Design review of the part built by this model. Coordinates are the model's own, in mm. Coordinates: 2 decimals unless noted, no trailing zeros. Loops run counter-clockwise (first coordinate to the right, second up) from the corner with the lowest first, then second, coordinate; pieces in that order, holes last. Notation, with made-up numbers: (68, -12.75) -> (110, -12.75) arc R22 cw to (110, 7.25) -> close; hole circle Ø6 at (-6, -17). An arc over 180 degrees is marked (long way). Use a Markdown table: item, result. Add a question column.
Q1. Take a section at D-D on z = 3. Write out the cut boundary in (x, y).
Q2. Take a section at B-B on x = -52.5. Write out the cut boundary in (y, z), plus the area to 3 significant figures.
Q3. Clearance check with a flat-ended pin moving along its axis: pin 1 Ø11.5 at (x, y) = (-50.8, 50.8) entering from -Z. State where the tip first meets the part, or that it passes through.
Q4. For probe 1 along Y at (x, z) = (-50.8, -3.5); probe 2 along X at (y, z) = (50.8, -20); probe 3 along Z at (x, y) = (6, 12), list the stretches that pass through material, from the lowest coordinate up.
Q5. Take a section at A-A on x = 0. Write out the cut boundary in (y, z).
Q6. Draft analysis for pull direction X (two halves, no side actions). For faces 1 (the face through (-1, 63.5, -13)), 2 (the face through (1, -1, -1.524)), 3 (the face through (63.5, -1, -14)), state which applies: pulls with the +X half, pulls with the -X half, needs draft (parallel to the pull), parting line crosses it, or undercut.
from build123d import *

# Parameters (mm, degrees)
F2_DEPTH = 63.5
F5_DEPTH = 50.8


with BuildPart() as f2:
    # F1 (on Front) → F2 (new body, symmetric)
    with BuildSketch(Plane.XZ):
        Polygon((-63.5, -32.291652), (63.5, -32.291652), (63.5, 5.808348), (0, 5.808348), (-63.5, 5.808348), align=None)
    extrude(amount=F2_DEPTH, both=True)

    # F0 (on Front) → F3 (revolve, cut)
    with BuildSketch(Plane.XZ):
        Polygon((38.1, -1.524), (50.8, 5.808348), (0, 5.808348), (0, -1.524), align=None)
    revolve(axis=Axis((0, 0, 2.142174), (0, 0, -1)), mode=Mode.SUBTRACT)

    # F4 (on Top) → F5 (cut, symmetric)
    with BuildSketch(Plane.XY):
        with BuildLine():
            ThreePointArc((-44.45, 50.8), (-55.290128, 55.290128), (-50.8, 44.45))
            Line((-50.8, 44.45), (-50.8, 50.8))
            Line((-50.8, 50.8), (-44.45, 50.8))
        make_face()
        with BuildLine():
            Line((-50.8, 50.8), (-50.8, 44.45))
            ThreePointArc((-50.8, 44.45), (-46.309872, 46.309872), (-44.45, 50.8))
            Line((-44.45, 50.8), (-50.8, 50.8))
        make_face()
    extrude(amount=F5_DEPTH, both=True, mode=Mode.SUBTRACT)


solid = f2.part
Answer list:
| question | item | result |
|---|---|---|
| 1 | outline | (-63.5, -63.5) -> (63.5, -63.5) -> (63.5, 63.5) -> (-63.5, 63.5) -> close; hole circle Ø12.7 at (-50.8, 50.8); hole circle Ø91.87 at (0, 0) |
| 2 | outline | (-63.5, -32.29) -> (44.68, -32.29) -> (44.68, 5.81) -> (-63.5, 5.81) -> close; (56.92, -32.29) -> (63.5, -32.29) -> (63.5, 5.81) -> (56.92, 5.81) -> close |
| 2 | area | 4,370 mm² |
| 3 | pin 1 | through |
| 4 | probe 1 | -63.5 to 44.45, 57.15 to 63.5 |
| 4 | probe 2 | -63.5 to -57.15, -44.45 to 63.5 |
| 4 | probe 3 | -32.29 to -1.52 |
| 5 | outline | (-63.5, -32.29) -> (63.5, -32.29) -> (63.5, 5.81) -> (50.8, 5.81) -> (38.1, -1.52) -> (-38.1, -1.52) -> (-50.8, 5.81) -> (-63.5, 5.81) -> close |
| 6 | face 1 | needs draft |
| 6 | face 2 | undercut |
| 6 | face 3 | pulls with the +X half |
